Design review of the part built by this model. Coordinates are the model's own, in mm. Face numbers are marked on the shaded views. A direction names the side the tool comes from. Coordinates: 2 decimals unless noted, no trailing zeros. Write each loop counter-clockwise with the first axis right and the second up, starting at its lowest first coordinate (ties: lowest second). Pieces come first, ordered by that corner, then holes.
Q1. Take a section at B-B, the plane y = 0.75. Write out the cut boundary in (x, z), plus the area to 3 significant figures.
Q2. For L1, parallel to Y at x = -1, z = 0.95; L2, parallel to Y at x = 3.5, z = -1.1; L3, parallel to X at y = 1.25, z = -1.25, list the stretches that pass through material, from the lowest coordinate up.
Q3. Take a section at D-D, the plane y = 3.5. Write out the cut boundary in (x, z).
Q4. The part is to be moulded in two halves that separate along X. For the marked faces 1, 2 and 3, say which applies: released by +X, released by -X, zero draft, split by the parting line, or undercut.
Q5. Take a section at A-A, the plane z = 0. Write out the cut boundary in (x, y), plus the area to 3 significant figures.
Q6. Take a section at C-C, the plane x = 26.5. Write out the cut boundary in (y, z).
Q7. For the marked faces 4, 5 and 6, list the 3-axis set-ups (+Z, -Z, +X, -X, +Y, -Y) from which the entire face can be reached by the end or side of a thin tool; tool diameter is ignored.
Q8. For pin 1 Ø1.5 at (x, z) = (0.5, -0.5) entering from -Y; pin 2 Ø5 at (x, y) = (21.5, 1.5) entering from +Z; pin 3 Ø3 at (y, z) = (0, 0.5) entering from +X; pin 4 Ø2 at (y, z) = (0, -0.5) entering from -X, all flat-tipped, find the tip position at first contact; note any pin that passes through.
from build123d import *

# Parameters (mm, degrees)
SKETCH1_R           = 1.5
BOSS_EXTRUDE1_DEPTH = 3
BOSS_EXTRUDE2_DEPTH = 2
SKETCH3_R           = 1.5
BOSS_EXTRUDE3_DEPTH = 7


with BuildPart() as part:
    # Sketch1 → Boss-Extrude1 (new body)
    with BuildSketch(Plane(origin=(0, 0, 0), x_dir=(1, 0, 0), z_dir=(0, 1, 0))):
        with Locations(Location((0, 0, 0), (0, 0, 270))):
            Circle(SKETCH1_R)
    extrude(amount=BOSS_EXTRUDE1_DEPTH)

    # Sketch2 → Boss-Extrude2 (add)
    with BuildSketch(Plane(origin=(0, 3, 0), x_dir=(1, 0, 0), z_dir=(0, 1, 0))):
        with BuildLine():
            Line((0, 2.75), (26, 2.75))
            ThreePointArc((26, 2.75), (28.75, 0), (26, -2.75))
            Line((26, -2.75), (0, -2.75))
            ThreePointArc((0, -2.75), (-2.75, 0), (0, 2.75))
        make_face()
    extrude(amount=BOSS_EXTRUDE2_DEPTH)

    # Sketch3 → Boss-Extrude3 (add)
    with BuildSketch(Plane.XZ.offset(-3)):
        with Locations(Location((26, 0, 0), (0, 0, 90))):
            Circle(SKETCH3_R)
    extrude(amount=BOSS_EXTRUDE3_DEPTH)


solid = part.part
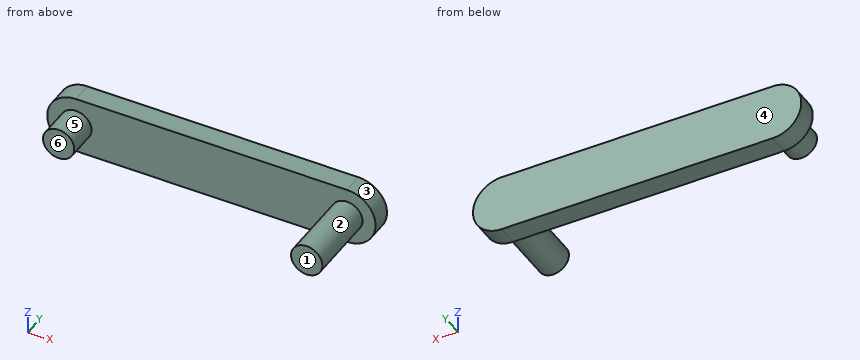
Responses:
1. outline: circle Ø3 at (0, 0); circle Ø3 at (26, 0)
1. area: 14.1 mm2
2. L1: y = 0 to 5
2. L2: y = 3 to 5
2. L3: x = -0.83 to 0.83, 25.17 to 26.83
3. outline: (0, -2.75) - (26, -2.75) arc R2.75 ccw to (26, 2.75) - (0, 2.75) arc R2.75 ccw to start
4. face 1: zero draft
4. face 2: undercut
4. face 3: released by +X
5. outline: (-2.75, 3) - (-1.5, 3) - (-1.5, 0) - (1.5, 0) - (1.5, 3) - (24.5, 3) - (24.5, -4) - (27.5, -4) - (27.5, 3) - (28.75, 3) - (28.75, 5) - (-2.75, 5) - close
5. area: 93.0 mm2
6. outline: (-4, -1.41) - (3, -1.41) - (3, -2.7) - (5, -2.7) - (5, 2.7) - (3, 2.7) - (3, 1.41) - (-4, 1.41) - close
7. face 4: +Z, -Z, +X, -X, +Y
7. face 5: -Y
7. face 6: +Z, -Z, -X, -Y
8. pin 1: stops at y = 0
8. pin 2: stops at z = 2.75
8. pin 3: stops at x = 27.5
8. pin 4: stops at x = -1.5
